Geometry check sheet. Reference: the model listing, model coordinates, mm. A direction names the side the tool comes from. Give positions to 0.01 mm unless a question says otherwise; leave off trailing zeros. Write each loop counter-clockwise with the first axis right and the second up, starting at its lowest first coordinate (ties: lowest second). Pieces come first, ordered by that corner, then holes.
(1) Cross-section at B-B (z = 0). Record the boundary of the cut face in (x, y) (3 decimals), and give its area (3 significant figures).
(2) Cross-section at D-D (x = 30.65). Record the boundary of the cut face in (y, z) (3 decimals).
(3) Thickness scan on line 1 along X through (y, z) = (2.6, -15.5); line 2 along X through (y, z) = (6.75, 5); line 3 along X through (y, z) = (1.5, 0). Record the ranges inside material, lowest first.
(4) Depth check by flat-ended pin: P1, Ø12, axis at x = 35, z = -3.5, coming from the -Y side; P2, Ø1, axis at y = 3, z = 10.5, coming from the -X side; P3, Ø4.5, axis at y = 3.5, z = -1, coming from the +X side. Enter the tip coordinate at first touch or a pass-through.
(5) Tool access check on faces 1 (the cylindrical face through (-39.02, 10.97, 6.99)), 2 (the flat face through (0, 4, 0)), 3 (the cylindrical face through (39.02, 10.97, 6.99)), 4 (the flat face through (-25.15, 5, 0)), 5 (the flat face through (25.15, 4, 0)). Record the directions out of +Z, -Z, +X, -X, +Y, -Y that give a thin tool (end or side, any length) a straight path to the whole face; none if there is none.
(6) Cross-section at A-A (y = 11.75). Record the boundary of the cut face in (x, z).
(7) Cross-section at C-C (x = -15.5). Record the boundary of the cut face in (y, z).
(8) Mould release check, pull along Z, two halves, no side actions. Record for faces 6 (the flat face through (-26.815, 9.48, -17.08)), 7 (the flat face through (-34, 9, 0)), 8 (the cylindrical face through (-32.796, 10.96, -0.676)): +Z half, -Z half, draft (parallel to the pull), parting line (faces both ways), or undercut.
```python
from build123d import *

# Parameters (mm, degrees)
SCHIZZO1_W                     = 50.3
SCHIZZO1_H                     = 42.3
ESTRUSIONE_ESTRUSIONE1_DEPTH   = 4
ESTRUSIONE_ESTRUSIONE2_DEPTH   = 42.3
SCHIZZO4_R                     = 2.25
TAGLIO_ESTRUSIONE1_DEPTH       = 42.3
FORO_PER_VITE_M4_1_D           = 4.5
FORO_PER_VITE_M4_1_DEPTH       = 4
FORO_PER_VITE_M4_1_CSINK_D     = 4.55
FORO_PER_VITE_M4_1_CSINK_ANGLE = 90
FORO_PER_VITE_M4_1_TIP         = 1.351936393
TAGLIO_ESTRUSIONE2_DEPTH       = 42.3
RACCORDO1_R                    = 10


with BuildPart() as part:
    # Schizzo1 → Estrusione-Estrusione1 (new body)
    with BuildSketch(Plane(origin=(0, 0, 0), x_dir=(1, 0, 0), z_dir=(0, 1, 0))):
        Rectangle(SCHIZZO1_W, SCHIZZO1_H)
    extrude(amount=ESTRUSIONE_ESTRUSIONE1_DEPTH)

    # Schizzo3 → Estrusione-Estrusione2 (add)
    with BuildSketch(Plane.XY.offset(21.15)):
        Polygon((-21.15, 4), (-21.15, 13), (-40.15, 13), (-40.15, 9), (-25.15, 9), (-25.15, 4), align=None)
        Polygon((25.15, 4), (25.15, 9), (40.15, 9), (40.15, 13), (21.15, 13), (21.15, 4), align=None)
    extrude(amount=-ESTRUSIONE_ESTRUSIONE2_DEPTH)

    # Schizzo4 → Taglio-Estrusione1 (cut)
    with BuildSketch(Plane(origin=(0, 4, 0), x_dir=(1, 0, 0), z_dir=(0, 1, 0))):
        with Locations(Location((-15.5, 15.5, 0), (0, 0, 270))):
            Circle(SCHIZZO4_R)
        with Locations(Location((15.5, 15.5, 0), (0, 0, 270))):
            Circle(SCHIZZO4_R)
        with Locations(Location((15.5, -15.5, 0), (0, 0, 270))):
            Circle(SCHIZZO4_R)
        with Locations(Location((-15.5, -15.5, 0), (0, 0, 270))):
            Circle(SCHIZZO4_R)
    extrude(amount=-TAGLIO_ESTRUSIONE1_DEPTH, mode=Mode.SUBTRACT)

    # Foro per Vite M4-1
    with Locations(Plane(origin=(0, 13, 0), x_dir=(1, 0, 0), z_dir=(0, 1, 0))):
        with Locations((-30.65, 0), (30.65, 0)):
            CounterSinkHole(FORO_PER_VITE_M4_1_D / 2, FORO_PER_VITE_M4_1_CSINK_D / 2, depth=FORO_PER_VITE_M4_1_DEPTH, counter_sink_angle=FORO_PER_VITE_M4_1_CSINK_ANGLE)
            with Locations((0, 0, -(FORO_PER_VITE_M4_1_DEPTH + FORO_PER_VITE_M4_1_TIP / 2))):  # 118° drill point
                Cone(0, FORO_PER_VITE_M4_1_D / 2, FORO_PER_VITE_M4_1_TIP, mode=Mode.SUBTRACT)

    # Schizzo7 → Taglio-Estrusione2 (cut)
    with BuildSketch(Plane(origin=(0, 13, 0), x_dir=(1, 0, 0), z_dir=(0, 1, 0))):
        Polygon((-21.15, -21.15), (-40.15, -7.5), (-40.15, -21.15), align=None)
        Polygon((-21.15, 21.15), (-40.15, 7.5), (-40.15, 21.15), align=None)
        Polygon((21.15, 21.15), (40.15, 21.15), (40.15, 7.5), align=None)
        Polygon((21.15, -21.15), (40.15, -21.15), (40.15, -7.5), align=None)
    extrude(amount=-TAGLIO_ESTRUSIONE2_DEPTH, mode=Mode.SUBTRACT)

    # Raccordo1
    raccordo1_edges = [part.edges().sort_by_distance(p)[0] for p in [
        (40.15, 11, 7.5),
        (40.15, 11, -7.5),
        (-40.15, 11, -7.5),
        (-40.15, 11, 7.5),
    ]]
    fillet(raccordo1_edges, radius=RACCORDO1_R)


solid = part.part
```
Reply:
1. outline: (-40.15, 9) - (-32.9, 9) - (-32.9, 12.975) - (-32.925, 13) - (-40.15, 13) - close; (-28.4, 9) - (-25.15, 9) - (-25.15, 0) - (25.15, 0) - (25.15, 9) - (28.4, 9) - (28.4, 12.975) - (28.375, 13) - (21.15, 13) - (21.15, 4) - (-21.15, 4) - (-21.15, 13) - (-28.375, 13) - (-28.4, 12.975) - close; (32.9, 9) - (40.15, 9) - (40.15, 13) - (32.925, 13) - (32.9, 12.975) - close
1. area: 357 mm2
2. outline: (9, -14.325) - (13, -14.325) - (13, -2.275) - (12.975, -2.25) - (9, -2.25) - close; (9, 2.25) - (12.975, 2.25) - (13, 2.275) - (13, 14.325) - (9, 14.325) - close
3. line 1: x = -25.15 to -17.75, -13.25 to 13.25, 17.75 to 25.15
3. line 2: x = -25.15 to -21.15, 21.15 to 25.15
3. line 3: x = -25.15 to 25.15
4. P1: stops at y = 9
4. P2: stops at x = -25.15
4. P3: stops at x = 25.15
5. face 1: +Z, -X, +Y, -Y
5. face 2: +Z, -Z, +Y
5. face 3: +Z, +X, +Y, -Y
5. face 4: +Z, -Z, -X, -Y
5. face 5: +Z, -Z, +X, -Y
6. outline: (-40.15, -2.37) arc R10 ccw to (-35.98, -10.49) - (-21.15, -21.15) - (-21.15, 21.15) - (-35.98, 10.49) arc R10 ccw to (-40.15, 2.37) - close; (21.15, -21.15) - (35.98, -10.49) arc R10 ccw to (40.15, -2.37) - (40.15, 2.37) arc R10 ccw to (35.98, 10.49) - (21.15, 21.15) - close; hole circle Ø4.5 at (-30.65, 0); hole circle Ø4.5 at (30.65, 0)
7. outline: (0, -21.15) - (4, -21.15) - (4, -17.75) - (0, -17.75) - close; (0, -13.25) - (4, -13.25) - (4, 13.25) - (0, 13.25) - close; (0, 17.75) - (4, 17.75) - (4, 21.15) - (0, 21.15) - close
8. face 6: -Z half
8. face 7: draft
8. face 8: undercut
